from build123d import *

# Parameters (mm, degrees)
F1_DEPTH = 2.54
F2_W     = 2.54
F2_H     = 110
F3_DEPTH = 2.54


with BuildPart() as f1:
    # F0 (on Front) → F1 (new body)
    with BuildSketch(Plane.XZ):
        Polygon((-20, -25), (20, -25), (20, 25), (0, 85), (-20, 85), (-20, 25), align=None)
    extrude(amount=F1_DEPTH)

    # F2 (on face) → F3 (join)
    with BuildSketch(Plane(origin=(-20, 0, 0), x_dir=(0, -1, 0), z_dir=(-1, 0, 0))):
        Polygon((-40, -25), (0, -25), (0, 85), (-20, 85), (-40, 30), align=None)
        with Locations((1.27, 30)):
            Rectangle(F2_W, F2_H)
    extrude(amount=F3_DEPTH)


solid = f1.part
The listing builds one solid part. Answer for the finished solid, in the listing's coordinates (mm). A direction names the side the tool comes from. Coordinates: 2 decimals unless noted, no trailing zeros. Order: outer loops, then holes, each group sorted by start corner. A loop starts at its lowest first (then second) coordinate and runs counter-clockwise, first axis right, second up. Notation, with made-up numbers: (-29.5, -33.5) -> (14.5, -33.5) arc R14 ccw to (14.5, -27.5) -> close; hole circle Ø10 at (60, 45.25). An arc over 180 degrees is marked (long way). Answer in a Markdown table with one row per item. Add a question column.
Item 1: Find section B-B (x = 11). Write down the section's boundary in (y, z), then the cut area to 3 significant figures.
Item 2: Which of the six approach directions +Z, -Z, +X, -X, +Y, -Y give full straight-line access (tool end or side, diameter ignored) to faces 1 (the face through (-20.4, 3.7, 85)), 2 (the face through (-20, 20, 31))?
Item 3: Find the intervals of material crossed by L1, parallel to Y at x = -6.5, z = 26; L2, parallel to X at y = 6, z = 40, in increasing order. Write a range as from..to.
Item 4: Find section A-A (z = 15). Write down the section's boundary in (x, y), then the cut area to 3 significant figures.
Item 5: Each of these flat-tipped pins is pushed along its axis until it touches: P1, Ø12, axis at x = 8, z = 16.5, coming from the +Y side; P2, Ø6, axis at y = 11, z = 17, coming from the +X side. Where does it stop, or does it pass through?
Item 6: Find section C-C (y = 25). Write down the section's boundary in (x, z), then the cut area to 3 significant figures.
Item 7: Find section D-D (z = 73). Write down the section's boundary in (x, y).
Result set:
| question | item | result |
|---|---|---|
| 1 | outline | (-2.54, -25) -> (0, -25) -> (0, 52) -> (-2.54, 52) -> close |
| 1 | area | 196 mm² |
| 2 | face 1 | +Z, +X, -X, +Y, -Y |
| 2 | face 2 | +Z, -Z, +X, +Y |
| 3 | L1 | y = -2.54..0 |
| 3 | L2 | x = -22.54..-20 |
| 4 | outline | (-22.54, -2.54) -> (20, -2.54) -> (20, 0) -> (-20, 0) -> (-20, 40) -> (-22.54, 40) -> close |
| 4 | area | 210 mm² |
| 5 | P1 | stops at y = 0 |
| 5 | P2 | stops at x = -20 |
| 6 | outline | (-22.54, -25) -> (-20, -25) -> (-20, 71.25) -> (-22.54, 71.25) -> close |
| 6 | area | 244 mm² |
| 7 | outline | (-22.54, -2.54) -> (4, -2.54) -> (4, 0) -> (-20, 0) -> (-20, 24.36) -> (-22.54, 24.36) -> close |
